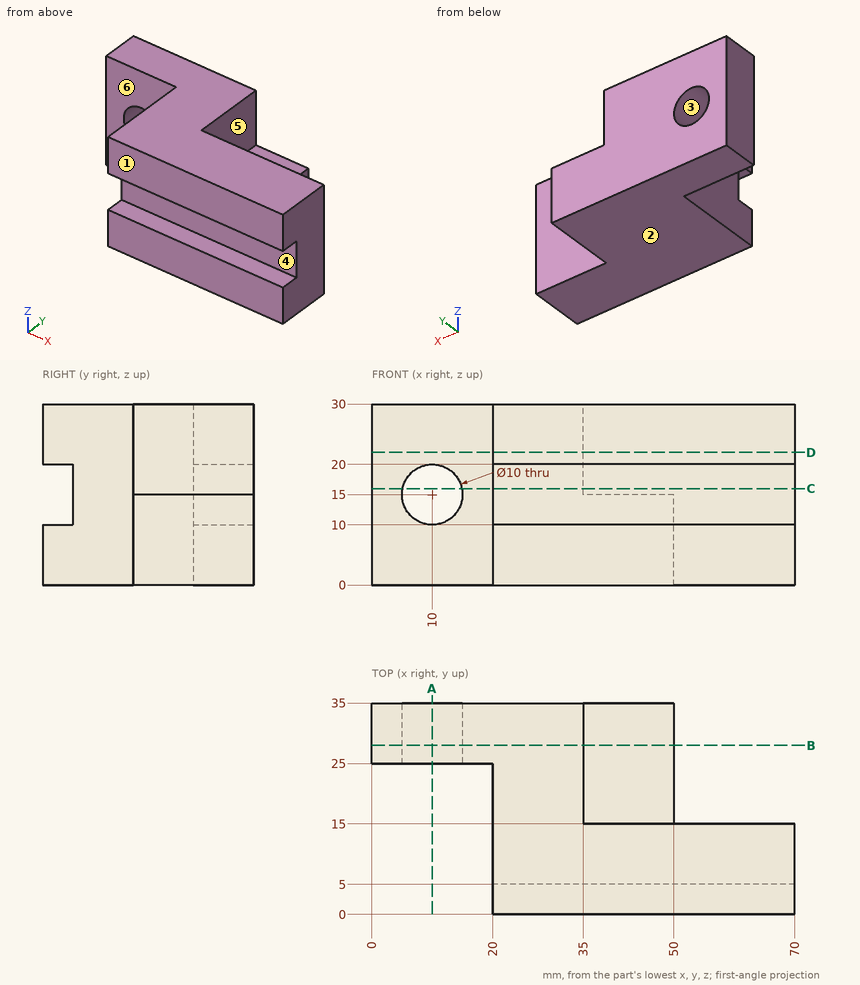
Geometry: see drawing. Coordinates: mm, zero at the bounding-box minimum. A direction names the side the tool comes from. Coordinates: 2 decimals unless noted, no trailing zeros. Loops run counter-clockwise (first coordinate to the right, second up) from the corner with the lowest first, then second, coordinate; pieces in that order, holes last. Notation, with made-up numbers: (-29, 71) - (-24, 71) arc R20 cw to (-24, 89) - close; hole circle Ø7 at (43, -15.5). An arc over 180 degrees is marked (long way). Put each result on its own line as item: value. Start each with the question number.
Q1. Cut plane C-C, the plane z = 16. Return loops of the section in (x, y), and give its area (3 significant figures).
Q2. Cut plane B-B, the plane y = 28. Return loops of the section in (x, z), and give its area (3 significant figures).
Q3. Pull-direction query (Z, two-part tool) for the marked faces 1, 2 and 3; classes: released by +Z, released by -Z, zero draft, split by the parting line, or undercut.
Q4. Cut plane D-D, the plane z = 22. Return loops of the section in (x, y), and give its area (3 significant figures).
Q5. Cut plane A-A, the plane x = 10. Return loops of the section in (y, z), and give its area (3 significant figures).
Q6. Line query: line 1 (Z direction, x = 10, y = 30.75); line 2 (Y direction, x = 64.5, z = 25.75). Output: solid intervals per line, ascending.
Q7. Set-up query: the marked faces 4, 5 and 6. Return all of +Z, -Z, +X, -X, +Y, -Y with unobstructed straight access to the full face (end or side cutting, diameter ignored); none if empty.
Q8. Pin query (flat end, axial travel): pin 1 Ø12.5 at (y, z) = (8.5, 8) entering from -X; pin 2 Ø15 at (x, z) = (53, 15) entering from +Y; pin 3 Ø6 at (x, y) = (48.5, 31) entering from +Z; pin 4 Ø7.5 at (y, z) = (28.5, 21.5) entering from +X. Return the tip coordinate at first contact, or that it passes through.
Filled sheet:
1. outline: (0, 25) - (5.1, 25) - (5.1, 35) - (0, 35) - close; (14.9, 25) - (20, 25) - (20, 5) - (70, 5) - (70, 15) - (35, 15) - (35, 35) - (14.9, 35) - close
1. area: 902 mm²
2. outline: (0, 0) - (50, 0) - (50, 15) - (35, 15) - (35, 30) - (0, 30) - close; hole circle Ø10 at (10, 15)
2. area: 1,200 mm²
3. face 1: zero draft
3. face 2: released by -Z
3. face 3: undercut
4. outline: (0, 25) - (20, 25) - (20, 0) - (70, 0) - (70, 15) - (35, 15) - (35, 35) - (0, 35) - close
4. area: 1,250 mm²
5. outline: (25, 0) - (35, 0) - (35, 10) - (25, 10) - close; (25, 20) - (35, 20) - (35, 30) - (25, 30) - close
5. area: 200 mm²
6. line 1: 0 to 10, 20 to 30
6. line 2: 0 to 15
7. face 4: +X, -X, -Y
7. face 5: +Z, +X, +Y
7. face 6: +Z, -Z, -X, -Y
8. pin 1: x = 20
8. pin 2: y = 35
8. pin 3: z = 15
8. pin 4: x = 35
